from build123d import *

# Parameters (mm, degrees)
SKETCH1_R                    = 6.35
BOSS_EXTRUDE1_DEPTH          = 21.844
SKETCH4_W                    = 4.630102794
SKETCH4_H                    = 9.398
SKETCH4_W_2                  = 5.584398789
CUT_EXTRUDE5_DEPTH           = 13.7
M5X0_8_TAPPED_HOLE2_D        = 4.2
F_5_16_24_TAPPED_HOLE1_D     = 6.9088
F_5_16_24_TAPPED_HOLE1_DEPTH = 6.35
F_5_16_24_TAPPED_HOLE1_TIP   = 2.075612922


with BuildPart() as part:
    # Sketch1 → Boss-Extrude1 (new body)
    with BuildSketch(Plane(origin=(0, 0, 0), x_dir=(1, 0, 0), z_dir=(0, 1, 0))):
        Circle(SKETCH1_R)
    extrude(amount=-BOSS_EXTRUDE1_DEPTH)

    # Sketch4 → Cut-Extrude5 (cut, through all)
    with BuildSketch(Plane(origin=(0, 0, -6.35), x_dir=(-1, 0, 0), z_dir=(0, 0, -1))):
        with Locations((-7.649051397, -10.922)):
            Rectangle(SKETCH4_W, SKETCH4_H)
        with Locations((8.126199395, -10.922)):
            Rectangle(SKETCH4_W_2, SKETCH4_H)
    extrude(amount=-CUT_EXTRUDE5_DEPTH, mode=Mode.SUBTRACT)

    # M5x0.8 Tapped Hole2 (through all)
    with Locations(Plane(origin=(0, 0, 0), x_dir=(1, 0, 0), z_dir=(0, 1, 0))):
        with Locations((0, 0)):
            Hole(M5X0_8_TAPPED_HOLE2_D / 2)

    # 5/16-24 Tapped Hole1
    with Locations(Plane(origin=(0, 0, 0), x_dir=(1, 0, 0), z_dir=(0, 1, 0))):
        with Locations((0, 0)):
            Hole(F_5_16_24_TAPPED_HOLE1_D / 2, depth=F_5_16_24_TAPPED_HOLE1_DEPTH)
            with Locations((0, 0, -(F_5_16_24_TAPPED_HOLE1_DEPTH + F_5_16_24_TAPPED_HOLE1_TIP / 2))):  # 118° drill point
                Cone(0, F_5_16_24_TAPPED_HOLE1_D / 2, F_5_16_24_TAPPED_HOLE1_TIP, mode=Mode.SUBTRACT)


solid = part.part
Read the model definition and answer for the solid it produces. Units are mm, in the model's axes. A direction names the side the tool comes from. Give positions to 0.01 mm unless a question says otherwise; leave off trailing zeros. Loops run counter-clockwise (first coordinate to the right, second up) from the corner with the lowest first, then second, coordinate; pieces in that order, holes last. Notation, with made-up numbers: (20.5, 4.5) - (53.5, 4.5) arc R29 ccw to (53.5, 26.5) - close; hole circle Ø2 at (-34, 61.25). An arc over 180 degrees is marked (long way). Answer as CSV lines item,"result". Start each with the question number.
1) Determine the mould class of faces 4 (the face through (0.45, -3.219, -3.425)), 5 (the face through (-4.68, -10.77, -4.29)), 6 (the face through (6, -6.223, 0)) for opening direction Z: released by +Z, released by -Z, zero draft, split by the parting line, or undercut.
2) Straight lines are drawn through the part: L1, parallel to Z at x = 0, y = -14.5; L2, parallel to Z at x = 0, y = -1.5; L3, parallel to Y at x = -5.5, z = -3. For each, find the intervals that lie inside material, in ascending order. Write a range as from..to.
3) Each of these flat-tipped pins is pushed along its axis until it touches: pin 1 Ø2 at (x, y) = (0.5, -6.5) entering from +Z; pin 2 Ø3 at (x, y) = (-2, -18.5) entering from -Z; pin 3 Ø3.5 at (x, z) = (0, 0) entering from -Y; pin 4 Ø4 at (y, z) = (-6.5, -2.5) entering from +X. Where does it stop, or does it pass through?
4) Find section A-A (z = 0). Write down the section's boundary in (x, y), then the cut area to 3 significant figures.
5) Find section C-C (y = -11.5). Write down the section's boundary in (x, z).
6) Find section B-B (x = 0). Write down the section's boundary in (y, z).
7) Find section D-D (y = -18.25). Write down the section's boundary in (x, z), then the cut area to 3 significant figures.
8) Which of the six approach directions +Z, -Z, +X, -X, +Y, -Y give full straight-line access (tool end or side, diameter ignored) to faces 1 (the face through (6, -15.621, 0)), 2 (the face through (-6, -15.621, 0)), 3 (the face through (-2.003, -14.607, -0.631))?
Findings below:
1,face 4,"undercut"
1,face 5,"split by the parting line"
1,face 6,"zero draft"
2,L1,"-6.35..-2.1, 2.1..6.35"
2,L2,"-6.35..-3.45, 3.45..6.35"
2,L3,"-21.84..-15.62, -6.22..0"
3,pin 1,"z = 6.35"
3,pin 2,"z = -6.33"
3,pin 3,"through"
3,pin 4,"x = 6.33"
4,outline,"(-6.35, -21.84) - (-2.1, -21.84) - (-2.1, -7.16) - (-3.45, -6.35) - (-3.45, 0) - (-6.35, 0) - (-6.35, -6.22) - (-5.33, -6.22) - (-5.33, -15.62) - (-6.35, -15.62) - close; (2.1, -21.84) - (6.35, -21.84) - (6.35, -15.62) - (5.33, -15.62) - (5.33, -6.22) - (6.35, -6.22) - (6.35, 0) - (3.45, 0) - (3.45, -6.35) - (2.1, -7.16) - close"
4,area,"148 mm^2"
5,outline,"(-5.33, -3.45) arc R6.35 ccw to (5.33, -3.45) - (5.33, 3.45) arc R6.35 ccw to (-5.33, 3.45) - close; hole circle Ø4.2 at (0, 0)"
6,outline,"(-21.84, -6.35) - (0, -6.35) - (0, -3.45) - (-6.35, -3.45) - (-7.16, -2.1) - (-21.84, -2.1) - close; (-21.84, 2.1) - (-7.16, 2.1) - (-6.35, 3.45) - (0, 3.45) - (0, 6.35) - (-21.84, 6.35) - close"
7,outline,"circle Ø12.7 at (0, 0); hole circle Ø4.2 at (0, 0)"
7,area,"113 mm^2"
8,face 1,"+Z, -Z, +X"
8,face 2,"+Z, -Z, -X"
8,face 3,"+Y, -Y"
